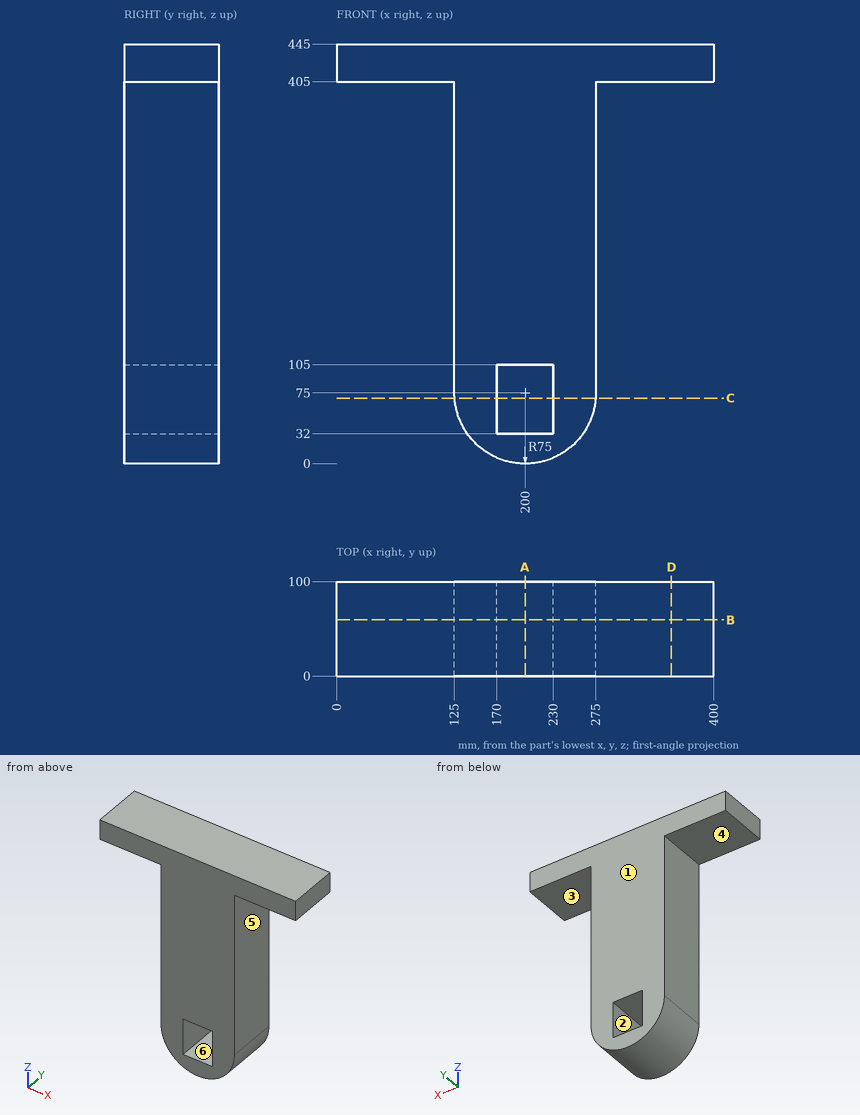
Design review of the part shown in the three views and the two pictorial views. Dimensions are in mm from the part's minimum x, y and z. A direction names the side the tool comes from. Round coordinates to 2 decimals unless told otherwise and drop trailing zeros. Write each loop counter-clockwise with the first axis right and the second up, starting at its lowest first coordinate (ties: lowest second). Pieces come first, ordered by that corner, then holes.
Item 1: We need section C-C on z = 69.5. Write out the cut boundary in (x, y).
Item 2: We need section D-D on x = 355. Write out the cut boundary in (y, z), and give its area (3 significant figures).
Item 3: We need section B-B on y = 59.5. Write out the cut boundary in (x, z).
Item 4: For the marked faces 4, 5 and 6, list the 3-axis set-ups (+Z, -Z, +X, -X, +Y, -Y) from which the entire face can be reached by the end or side of a thin tool; tool diameter is ignored.
Item 5: For probe 1 along X at (y, z) = (54.5, 94); probe 2 along X at (y, z) = (63, 333); probe 3 along Z at (x, y) = (112.5, 79), list the stretches that pass through material, from the lowest coordinate up.
Item 6: We need section A-A on x = 200. Write out the cut boundary in (y, z), and give its area (3 significant figures).
Item 7: The part is to be moulded in two halves that separate along Z. For the marked faces 1, 2 and 3, say which applies: +Z half, -Z half, draft (parallel to the pull), parting line (faces both ways), or undercut.
Item 8: Clearance check with flat-ended pins moving along their axes: pin 1 Ø4 at (x, y) = (271.5, 23.5) entering from -Z; pin 2 Ø22 at (y, z) = (27, 62.5) entering from -X (3 decimals); pin 3 Ø4 at (x, y) = (58, 27) entering from -Z. State where each tip first meets the part, or that it passes through.
Returned:
1. outline: (125.2, 0) - (170, 0) - (170, 100) - (125.2, 100) - close; (230, 0) - (274.8, 0) - (274.8, 100) - (230, 100) - close
2. outline: (0, 405) - (100, 405) - (100, 445) - (0, 445) - close
2. area: 4,000 mm2
3. outline: (0, 405) - (125, 405) - (125, 75) arc R75 ccw to (275, 75) - (275, 405) - (400, 405) - (400, 445) - (0, 445) - close; hole (170, 32) - (230, 32) - (230, 105) - (170, 105) - close
4. face 4: -Z, -X, +Y, -Y
4. face 5: -Z, +X, +Y, -Y
4. face 6: +Y, -Y
5. probe 1: x = 125 to 170, 230 to 275
5. probe 2: x = 125 to 275
5. probe 3: z = 405 to 445
6. outline: (0, 0) - (100, 0) - (100, 32) - (0, 32) - close; (0, 105) - (100, 105) - (100, 445) - (0, 445) - close
6. area: 37,200 mm2
7. face 1: draft
7. face 2: undercut
7. face 3: -Z half
8. pin 1: stops at z = 46.81
8. pin 2: stops at x = 125.015
8. pin 3: stops at z = 405
